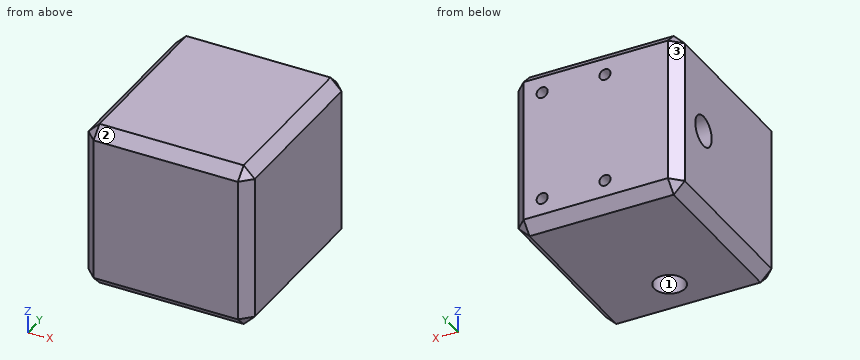
```python
from build123d import *

# Parameters (mm, degrees)
SKETCH1_W           = 45
SKETCH1_H           = 45
BOSS_EXTRUDE1_DEPTH = 50
SKETCH2_R           = 4.15
CUT_EXTRUDE1_DEPTH  = 30
SKETCH3_R           = 4.15
CUT_EXTRUDE2_DEPTH  = 30
CHAMFER1_SIZE       = 3
SKETCH5_R           = 1.5
CUT_EXTRUDE3_DEPTH  = 10


with BuildPart() as part:
    # Sketch1 → Boss-Extrude1 (new body)
    with BuildSketch(Plane(origin=(0, 0, 0), x_dir=(1, 0, 0), z_dir=(0, 1, 0))):
        Rectangle(SKETCH1_W, SKETCH1_H)
    extrude(amount=BOSS_EXTRUDE1_DEPTH)

    # Sketch2 → Cut-Extrude1 (cut)
    with BuildSketch(Plane(origin=(0, 0, -22.5), x_dir=(-1, 0, 0), z_dir=(0, 0, -1))):
        with Locations((0, 12.5)):
            Circle(SKETCH2_R)
    extrude(amount=-CUT_EXTRUDE1_DEPTH, mode=Mode.SUBTRACT)

    # Sketch3 → Cut-Extrude2 (cut)
    with BuildSketch(Plane.ZY.offset(22.5)):
        with Locations((0, 37.5)):
            Circle(SKETCH3_R)
    extrude(amount=-CUT_EXTRUDE2_DEPTH, mode=Mode.SUBTRACT)

    # Chamfer1
    chamfer1_edges = [part.edges().sort_by_distance(p)[0] for p in [
        (-22.5, 50, 0),
        (0, 50, 22.5),
        (22.5, 50, 0),
        (0, 0, 22.5),
        (-22.5, 0, 0),
        (0, 0, -22.5),
        (22.5, 0, 0),
        (22.5, 25, 22.5),
        (-22.5, 25, 22.5),
        (-22.5, 25, -22.5),
        (22.5, 25, -22.5),
        (0, 50, -22.5),
    ]]
    chamfer(chamfer1_edges, length=CHAMFER1_SIZE)

    # Sketch5 → Cut-Extrude3 (cut)
    with BuildSketch(Plane(origin=(0, 50, 0), x_dir=(1, 0, 0), z_dir=(0, 1, 0))):
        with Locations(Location((-2.51, -15, 0), (0, 0, 270))):
            Circle(SKETCH5_R)
        with Locations(Location((14.49, -15, 0), (0, 0, 270))):
            Circle(SKETCH5_R)
        with Locations(Location((14.49, 15, 0), (0, 0, 90))):
            Circle(SKETCH5_R)
        with Locations(Location((-2.51, 15, 0), (0, 0, 90))):
            Circle(SKETCH5_R)
    extrude(amount=-CUT_EXTRUDE3_DEPTH, mode=Mode.SUBTRACT)


solid = part.part
```
Could you check a few things on this model? Use its own coordinates, in mm. Face numbers are marked on the shaded views. Coordinates: 2 decimals unless noted, no trailing zeros. Write each loop counter-clockwise with the first axis right and the second up, starting at its lowest first coordinate (ties: lowest second). Pieces come first, ordered by that corner, then holes. Notation, with made-up numbers: (-3.75, 65) -> (26.25, 65) arc R31 cw to (26.25, 98) -> close; hole circle Ø11 at (-33.5, -26). An arc over 180 degrees is marked (long way). Write item = value, one per line. Start each with the question number.
(1) Will these pins go through, and if not, where does the flat tip stop? pin 1 (2.5 mm diameter, centred on y = 35.5, z = 1.5, fed in from -X); pin 2 (5 mm diameter, centred on x = 0, y = 12.5, fed in from -Z); pin 3 (0.9 mm diameter, centred on x = 15, z = -15, fed in from +Y).
(2) I want a section at D-D (x = 14.49). Please give me the cut outline in (y, z), plus the area to 3 significant figures.
(3) I want a section at A-A (x = 0). Please give me the cut outline in (y, z), plus the area to 3 significant figures.
(4) I need wall thicknesses on line 1 (X direction, y = 47, z = 15); line 2 (Z direction, x = 13.5, y = 44); line 3 (Z direction, x = 14, y = 47). Which ranges of each line are inside material? Lowest first, please. Write a range as [from, to].
(5) We'd pull the mould along X, two halves only. Please class the marked faces 1, 2 and 3: released by +X, released by -X, zero draft, split by the parting line, or undercut.
(6) I want a section at C-C (y = 37.5). Please give me the cut outline in (x, z).
(7) I want a section at B-B (z = 0). Please give me the cut outline in (x, y), plus the area to 3 significant figures.
Result set:
q1.pin_1 = 7.5
q1.pin_2 = 7.5
q1.pin_3 = 40
q2.outline = (0, -19.5) -> (3, -22.5) -> (47, -22.5) -> (50, -19.5) -> (50, -16.5) -> (40, -16.5) -> (40, -13.5) -> (50, -13.5) -> (50, 13.5) -> (40, 13.5) -> (40, 16.5) -> (50, 16.5) -> (50, 19.5) -> (47, 22.5) -> (3, 22.5) -> (0, 19.5) -> close
q2.area = 2,170 mm2
q3.outline = (0, -19.5) -> (3, -22.5) -> (8.35, -22.5) -> (8.35, 7.5) -> (16.65, 7.5) -> (16.65, -22.5) -> (47, -22.5) -> (50, -19.5) -> (50, 19.5) -> (47, 22.5) -> (3, 22.5) -> (0, 19.5) -> close; hole circle Ø8.3 at (37.5, 0)
q3.area = 1,930 mm2
q4.line_1 = [-22.5, -4.01], [-1.01, 12.99], [15.99, 22.5]
q4.line_2 = [-22.5, -16.13], [-13.87, 13.87], [16.13, 22.5]
q4.line_3 = [-22.5, -16.42], [-13.58, 13.58], [16.42, 22.5]
q5.face_1 = undercut
q5.face_2 = zero draft
q5.face_3 = released by -X
q6.outline = (-22.5, -19.5) -> (-19.5, -22.5) -> (19.5, -22.5) -> (22.5, -19.5) -> (22.5, 19.5) -> (19.5, 22.5) -> (-19.5, 22.5) -> (-22.5, 19.5) -> (-22.5, 4.15) -> (7.5, 4.15) -> (7.5, -4.15) -> (-22.5, -4.15) -> close
q7.outline = (-22.5, 3) -> (-19.5, 0) -> (19.5, 0) -> (22.5, 3) -> (22.5, 47) -> (19.5, 50) -> (-19.5, 50) -> (-22.5, 47) -> (-22.5, 41.65) -> (7.5, 41.65) -> (7.5, 33.35) -> (-22.5, 33.35) -> close; hole circle Ø8.3 at (0, 12.5)
q7.area = 1,930 mm2
